Could you check a few things on this model? Use its own coordinates, in mm. A direction names the side the tool comes from. Give positions to 0.01 mm unless a question says otherwise; leave off trailing zeros. Loops run counter-clockwise (first coordinate to the right, second up) from the corner with the lowest first, then second, coordinate; pieces in that order, holes last. Notation, with made-up numbers: (33, 66.25) -> (89, 66.25) arc R27 ccw to (89, 98.25) -> close; hole circle Ø4 at (69.25, -8). An arc over 180 degrees is marked (long way). Write each question's results on one line, items separated by ' | '. Start each with the question number.
Q1. Will these pins go through, and if not, where does the flat tip stop? P1, Ø1, axis at x = -9.5, z = 0.5, coming from the +Y side; P2, Ø2, axis at x = -6, z = 0.5, coming from the -Y side; P3, Ø0.6, axis at x = 59, y = 0, coming from the +Z side.
Q2. If I drill on line 1 along Y through (x, z) = (22.5, 0.25); line 2 along Z through (x, y) = (14, 0.8), over which ranges is the centre line in solid material (lowest first)?
Q3. Which directions (+Z, -Z, +X, -X, +Y, -Y) give clear straight access to the entire face, cutting with the end or side of a thin tool? Please do faces 1 (the face through (-8, -0.25, 0)), 2 (the face through (60, -0.25, 0)), 3 (the face through (-8, 0.25, 0)), 4 (the face through (60, 0.25, 0)).
Q4. If we section it at A-A, the plane x = 27: List the corners of the cut face in (y, z) for me, plus the area to 3 significant figures.
from build123d import *

# Parameters (mm, degrees)
SKETCH_7_R      = 0.5
EXTRUDE_1_DEPTH = 57.8
SKETCH_8_W      = 2
SKETCH_8_H      = 0.5
EXTRUDE_2_DEPTH = 10
CHAMFER_1_SIZE  = 0.5
SKETCH_9_W      = 2
SKETCH_9_H      = 0.5
EXTRUDE_3_DEPTH = 10
CHAMFER_2_SIZE  = 0.5


with BuildPart() as part:
    # По траектории1: sweep along a path in Эскиз4
    with BuildLine(Plane(origin=(0, 0, 0), x_dir=(0, 0, -1), z_dir=(1, 0, 0))) as sweep_1_path:
        CenterArc((0, 0), 2.7, 0, 360)
    # Эскиз3 → По траектории1 (sweep)
    with BuildSketch(Plane(origin=(0, 0, 0), x_dir=(1, 0, 0), z_dir=(0, 1, 0))):
        with BuildLine():
            Line((48.854990775, 2.7), (49.31, 2.7))
            ThreePointArc((49.31, 2.7), (51.212117241, 1.912117241), (52, 0.01))
            Line((52, 0.01), (52, 0))
            Line((52, 0), (0, 0))
            Line((0, 0), (0, 0.01))
            ThreePointArc((0, 0.01), (0.787882759, 1.912117241), (2.69, 2.7))
            Line((2.69, 2.7), (3.145009225, 2.7))
            ThreePointArc((3.145009225, 2.7), (3.537804142, 2.671167442), (3.922178774, 2.585287846))
            ThreePointArc((3.922178774, 2.585287846), (4.5, 2.5), (5.077821226, 2.585287846))
            ThreePointArc((5.077821226, 2.585287846), (5.462195858, 2.671167442), (5.854990775, 2.7))
            Line((5.854990775, 2.7), (46.145009225, 2.7))
            ThreePointArc((46.145009225, 2.7), (46.537804142, 2.671167442), (46.922178774, 2.585287846))
            ThreePointArc((46.922178774, 2.585287846), (47.5, 2.5), (48.077821226, 2.585287846))
            ThreePointArc((48.077821226, 2.585287846), (48.462195858, 2.671167442), (48.854990775, 2.7))
        make_face()
    sweep(path=sweep_1_path.line)

    # Эскиз7 → Бобышка-Вытянуть1 (add)
    with BuildSketch(Plane(origin=(-2.9, 0, 0), x_dir=(0, 0, -1), z_dir=(1, 0, 0))):
        Circle(SKETCH_7_R)
    extrude(amount=EXTRUDE_1_DEPTH)

    # Эскиз8 → Бобышка-Вытянуть2 (add)
    with BuildSketch(Plane.ZY.offset(2.9)):
        Rectangle(SKETCH_8_W, SKETCH_8_H)
    extrude(amount=EXTRUDE_2_DEPTH)

    # Фаска1
    chamfer_1_edges = [part.edges().sort_by_distance(p)[0] for p in [
        (-2.9, 0, -1),
        (-2.9, 0, 1),
    ]]
    chamfer(chamfer_1_edges, length=CHAMFER_1_SIZE - 0.0001)  # a hair under: the kernel refuses the full size

    # Эскиз9 → Бобышка-Вытянуть3 (add)
    with BuildSketch(Plane(origin=(54.9, 0, 0), x_dir=(0, 0, -1), z_dir=(1, 0, 0))):
        Rectangle(SKETCH_9_W, SKETCH_9_H)
    extrude(amount=EXTRUDE_3_DEPTH)

    # Фаска2
    chamfer_2_edges = [part.edges().sort_by_distance(p)[0] for p in [
        (54.9, 0, -1),
        (54.9, 0, 1),
    ]]
    chamfer(chamfer_2_edges, length=CHAMFER_2_SIZE - 0.0001)  # a hair under: the kernel refuses the full size


solid = part.part
Final values:
1) P1: stops at y = 0.25 | P2: stops at y = -0.25 | P3: stops at z = 1
2) line 1: y = -2.69 to 2.69 | line 2: z = -2.58 to 2.58
3) face 1: +Z, -Z, -X, -Y | face 2: +Z, -Z, +X, -Y | face 3: +Z, -Z, -X, +Y | face 4: +Z, -Z, +X, +Y
4) outline: circle Ø5.4 at (0, 0) | area: 22.9 mm²
